The model under review builds one solid part; all positions refer to its coordinate system, in mm. A direction names the side the tool comes from. Give positions to 0.01 mm unless a question says otherwise; leave off trailing zeros. Order: outer loops, then holes, each group sorted by start corner. A loop starts at its lowest first (then second) coordinate and runs counter-clockwise, first axis right, second up. Notation, with made-up numbers: (-31.75, -16) - (-13.75, -16) arc R13 cw to (-13.75, -2) - close; hole circle Ø10 at (-21.75, -12). An arc over 180 degrees is marked (long way). Use CSV: the item, a comma, the result in double quotes.
```python
from build123d import *

# Parameters (mm, degrees)
F0_R      = 38.1
F1_DEPTH  = 76.2
F2_R      = 33.02
F3_DEPTH  = 69.85
F5_R      = 12.7
F6_DEPTH  = 127
F6_FACE_R = 12.7
F4_R      = 31.75
F8_R      = 43.18
F9_DEPTH  = 25.4


with BuildPart() as f1:
    # F0 (on Front) → F1 (new body)
    with BuildSketch(Plane.XZ):
        Circle(F0_R)
    extrude(amount=F1_DEPTH)

    # F2 (on face) → F3 (cut)
    with BuildSketch(Plane.XZ.offset(76.2)):
        Circle(F2_R)
    extrude(amount=-F3_DEPTH, mode=Mode.SUBTRACT)

    # F5 (on Front) → F6 (join)
    with BuildSketch(Plane.XZ):
        Circle(F5_R)
    extrude(amount=-F6_DEPTH)

    # F6_face (on face) → F7 section 0
    with BuildSketch(Plane(origin=(0, 127, 0), x_dir=(1, 0, 0), z_dir=(0, 1, 0))):
        Circle(F6_FACE_R)
    # F4 (on face) → F7 section 1
    with BuildSketch(Plane(origin=(0, 0, 0), x_dir=(-1, 0, 0), z_dir=(0, 1, 0))):
        Circle(F4_R)
    loft()

    # F8 (on Front) → F9 (join)
    with BuildSketch(Plane.XZ):
        Circle(F8_R)
    extrude(amount=F9_DEPTH)


solid = f1.part
```
Item 1: Clearance check with flat-ended pins moving along their axes: pin 1 (4 mm diameter, centred on y = 1.5, z = 12.5, fed in from -X); pin 2 (1 mm diameter, centred on y = 68, z = 11, fed in from -X); pin 3 (3 mm diameter, centred on y = 16, z = -7, fed in from +X). State where each tip first meets the part, or that it passes through.
Results list:
pin 1,"stops at x = -41.71"
pin 2,"stops at x = -18.83"
pin 3,"stops at x = 28.91"
Item 2: Take a section at A-A, the plane x = 0. Give the boundary of the cut face in (y, z).
Results list:
outline,"(-76.2, -38.1) - (-25.4, -38.1) - (-25.4, -43.18) - (0, -43.18) - (0, -31.75) - (127, -12.7) - (127, 12.7) - (0, 31.75) - (0, 43.18) - (-25.4, 43.18) - (-25.4, 38.1) - (-76.2, 38.1) - (-76.2, 33.02) - (-25.4, 33.02) - (-25.4, -33.02) - (-76.2, -33.02) - close"
Item 3: Wall thickness on L1, parallel to Z at x = 0, y = -48.5; L2, parallel to Y at x = -4, z = -37; L3, parallel to Y at x = 11, z = -1.5: over which ranges is each line inside the solid? List them lowest first.
Results list:
L1,"z = -38.1 to -33.02, 33.02 to 38.1"
L2,"y = -76.2 to 0"
L3,"y = -25.4 to 127"
Item 4: Tool access review of faces 4 (the face through (-31.83, -12.52, 29.18)), 5 (the face through (3, -25.4, -38.2)): name each direction out of +Z, -Z, +X, -X, +Y, -Y from which nothing blocks a thin tool from reaching the whole face with its end or side.
Results list:
face 4,"+Y, -Y"
face 5,"-Y"
Item 5: Take a section at B-B, the plane y = 103. Give the boundary of the cut face in (x, z), and give its area (3 significant figures).
Results list:
outline,"circle Ø32.6 at (0, 0)"
area,"835 mm2"
Item 6: Mouldability with a two-part tool opening along Z and no side actions: class faces 1 (the face through (0, -25.4, 0)), 2 (the face through (-30.235, -50.444, -23.183)), 3 (the face through (-23, 0, 23)) as pulls with the +Z half, pulls with the -Z half, needs draft (parallel to the pull), parting line crosses it, or undercut.
Results list:
face 1,"undercut"
face 2,"parting line crosses it"
face 3,"needs draft"
Item 7: Take a section at C-C, the plane y = 70. Give the boundary of the cut face in (x, z).
Results list:
outline,"circle Ø42.5 at (0, 0)"
